from build123d import *

# Parameters (mm, degrees)
BOSS_EXTRUDE1_DEPTH = 49.911
FILLET1_R           = 12.7


with BuildPart() as part:
    # Sketch1 → Boss-Extrude1 (new, symmetric)
    with BuildSketch(Plane(origin=(0, 0, 0), x_dir=(0, 0, -1), z_dir=(1, 0, 0))):
        Polygon((0, 0), (0, 55.88), (304.8, 55.88), (411.035788296, 1.516400562), (381.1016, 0), align=None)
    extrude(amount=BOSS_EXTRUDE1_DEPTH, both=True)

    # Fillet1
    # the kernel refuses this fillet: 12.7 mm, written as the material it takes off along each edge
    with BuildSketch(Plane(origin=(49.911, 0, -412.8516), x_dir=(0, 1, 0), z_dir=(0, 0, 1))) as fillet1_piece_1:
        with BuildLine():
            CenterArc((FILLET1_R, FILLET1_R), FILLET1_R, 180, 90)
            Line((0, FILLET1_R), (0, 0))
            Line((0, 0), (FILLET1_R, 0))
        make_face()
    extrude(amount=444.6016, mode=Mode.SUBTRACT)
    with BuildSketch(Plane(origin=(-49.911, 3.12272641, -442.745127887), x_dir=(1, 0, 0), z_dir=(0, -0.0505929400767125, 0.9987193571841863)), Plane(origin=(49.911, 3.12272641, -442.745127887), x_dir=(0, 0.9987193571841864, 0.0505929400767125), z_dir=(0, -0.0505929400767125, 0.9987193571841863))) as fillet1_piece_2:
        with BuildLine():
            CenterArc((FILLET1_R, FILLET1_R), FILLET1_R, 180, 90)
            Line((0, FILLET1_R), (0, 0))
            Line((0, 0), (FILLET1_R, 0))
        make_face()
    extrude(amount=93.472572456, mode=Mode.SUBTRACT)
    with BuildSketch(Plane(origin=(-49.911, 0, -412.8516), x_dir=(0, 1, 0), z_dir=(0, 0, 1))) as fillet1_piece_3:
        with BuildLine():
            CenterArc((FILLET1_R, -FILLET1_R), FILLET1_R, 90, 90)
            Line((0, -FILLET1_R), (0, 0))
            Line((0, 0), (FILLET1_R, 0))
        make_face()
    extrude(amount=444.6016, mode=Mode.SUBTRACT)


solid = part.part
Can you work these out from the model? Positions are in its coordinate system, mm. Coordinates: 2 decimals unless noted, no trailing zeros. Loops run counter-clockwise (first coordinate to the right, second up) from the corner with the lowest first, then second, coordinate; pieces in that order, holes last. Notation, with made-up numbers: (89.25, -36) - (98.25, -36) arc R11 cw to (98.25, -17) - close; hole circle Ø3 at (54.5, 28). An arc over 180 degrees is marked (long way). Put each result on its own line as item: value. Start each with the question number.
Item 1: If I drill on line 1 along Z through (x, y) = (36, 12); line 2 along Z through (x, y) = (32.5, 28.5); line 3 along Y through (x, z) = (25, -346), over which ranges is the centre line in solid material (lowest first)?
Item 2: For pin 1 (5 mm diameter, centred on x = 3, y = 31.5, fed in from -Z); pin 2 (12 mm diameter, centred on x = 27.5, y = 39.5, fed in from +Z); pin 3 (10 mm diameter, centred on y = 6, z = -332.5, fed in from -X), each with a flat end and sliding along its axis, tell me the tip position at first contact or that it passes through.
Item 3: Suppose I cut it at C-C (y = 38.5). Please give me the cut outline in (x, z).
Item 4: Suppose I cut it at B-B (z = -312). Please give me the cut outline in (x, y), and give its area (3 significant figures).
Item 5: Suppose I cut it at A-A (x = -23.5). Please give me the cut outline in (y, z), and give its area (3 significant figures).
Here are the results:
1. line 1: -390.55 to 0
1. line 2: -358.31 to 0
1. line 3: 0 to 34.8
2. pin 1: z = -357.33
2. pin 2: z = 0
2. pin 3: x = -49.8
3. outline: (-49.91, -338.76) - (49.91, -338.76) - (49.91, 0) - (-49.91, 0) - close
4. outline: (-49.91, 12.7) arc R12.7 ccw to (-37.21, 0) - (37.21, 0) arc R12.7 ccw to (49.91, 12.7) - (49.91, 52.2) - (-49.91, 52.2) - close
4. area: 5,140 mm²
5. outline: (0, -381.1) - (1.52, -411.04) - (55.88, -304.8) - (55.88, 0) - (0, 0) - close
5. area: 20,100 mm²
